For this review, take the finished solid that the model builds, in its own axes (mm). A direction names the side the tool comes from. Coordinates: 2 decimals unless noted, no trailing zeros. Order: outer loops, then holes, each group sorted by start corner. A loop starts at its lowest first (then second) coordinate and runs counter-clockwise, first axis right, second up. Notation, with made-up numbers: (-28.75, 75.25) - (-5.75, 75.25) arc R20 ccw to (-5.75, 112.25) - close; hole circle Ø7 at (38, 11). An arc over 180 degrees is marked (long way). One line per item, written item: value. Start each with the question number.
(1) Consider section A-A on z = -3.25. Write out the cut boundary in (x, y).
(2) Consider section D-D on x = -6.25. Write out the cut boundary in (y, z), then the cut area to 3 significant figures.
(3) Consider section C-C on z = -5.5. Write out the cut boundary in (x, y), then the cut area to 3 significant figures.
(4) Consider section B-B on y = -3.25. Write out the cut boundary in (x, z).
(5) For faces 1 (the flat face through (-7, 3, 6.17)), 2 (the flat face through (0, 0, 10.17)), 3 (the flat face through (-6.825, 1.144, 7.031)), 4 (the flat face through (6.775, 1.144, 7.031)), 5 (the flat face through (0, 2.671, -3)), list the 3-axis set-ups (+Z, -Z, +X, -X, +Y, -Y) from which the entire face can be reached by the end or side of a thin tool; tool diameter is ignored.
(6) To check wall thickness, follow line 1 along X through (y, z) = (-2.5, -6.5); line 2 along X through (y, z) = (2.5, 9); line 3 along Z through (x, y) = (-0.5, 3.75). State the ranges of each line that lie inside material, in increasing order.
(7) Clearance check with flat-ended pins moving along their axes: pin 1 (4 mm diameter, centred on y = 0.5, z = 4, fed in from +X); pin 2 (1 mm diameter, centred on x = -7.5, y = 3, fed in from -Z); pin 3 (8 mm diameter, centred on x = -1.5, z = -6, fed in from -Y). State where each tip first meets the part, or that it passes through.
(8) Mouldability with a two-part tool opening along Y and no side actions: class faces 6 (the flat face through (0, -2.329, -3)), 7 (the flat face through (0, 4.25, 5)), 8 (the flat face through (-3.836, 0, 10)), 9 (the flat face through (0, -1.791, 9)) as released by +Y, released by -Y, zero draft, split by the parting line, or undercut.
```python
from build123d import *

# Parameters (mm, degrees)
SKETCH1_W           = 10
SKETCH1_H           = 8.5
BOSS_EXTRUDE1_DEPTH = 10.67
SKETCH2_W           = 7.4
SKETCH2_H           = 0.5
BOSS_EXTRUDE2_DEPTH = 1.5
SKETCH3_W           = 2.8
SKETCH3_H           = 0.5
BOSS_EXTRUDE3_DEPTH = 7.06
FILLET4_R           = 0.1
SKETCH5_W           = 4.5
SKETCH5_H           = 8.5
BOSS_EXTRUDE4_DEPTH = 3.6
SKETCH6_W           = 4.5
SKETCH6_H           = 8.5
BOSS_EXTRUDE5_DEPTH = 3.6
CUT_EXTRUDE2_START  = -17.2
CUT_EXTRUDE2_DEPTH  = 17.2
BOSS_EXTRUDE6_DEPTH = 10
SKETCH9_W           = 15.5
SKETCH9_H           = 8.5
CUT_EXTRUDE3_DEPTH  = 2
SKETCH10_W          = 7.671768302
SKETCH10_H          = 3.58137051
BOSS_EXTRUDE7_DEPTH = 2
SKETCH12_W          = 7.671768302
SKETCH12_H          = 1.176323548
CUT_EXTRUDE4_DEPTH  = 0.5
FILLET7_R           = 1
FILLET8_R           = 0.5
SKETCH13_W          = 1.4
SKETCH13_H          = 3.317554906
CUT_EXTRUDE5_DEPTH  = 10
FILLET9_R           = 0.3


with BuildPart() as part:
    # Sketch1 → Boss-Extrude1 (new body)
    with BuildSketch(Plane.XY):
        Rectangle(SKETCH1_W, SKETCH1_H)
    extrude(amount=BOSS_EXTRUDE1_DEPTH)

    # Sketch2 → Boss-Extrude2 (add)
    with BuildSketch(Plane(origin=(0, 0, 0), x_dir=(-1, 0, 0), z_dir=(0, 0, -1))):
        with Locations((0.121950207, -2.578749491)):
            Rectangle(SKETCH2_W, SKETCH2_H)
        with Locations((0.121950207, 2.421250509)):
            Rectangle(SKETCH2_W, SKETCH2_H)
    extrude(amount=BOSS_EXTRUDE2_DEPTH)

    # Sketch3 → Boss-Extrude3 (add)
    with BuildSketch(Plane(origin=(0, 0, -1.5), x_dir=(-1, 0, 0), z_dir=(0, 0, -1))):
        with Locations((0, -2.578749491)):
            Rectangle(SKETCH3_W, SKETCH3_H)
        with Locations((0.006424345, 2.421250509)):
            Rectangle(SKETCH3_W, SKETCH3_H)
    extrude(amount=BOSS_EXTRUDE3_DEPTH)

    # Fillet4
    fillet4_edges = [part.edges().sort_by_distance(p)[0] for p in [
        (2.489024896, -2.828749491, -1.5),
        (-2.610975104, -2.328749491, -1.5),
        (-2.614187276, 2.671250509, -1.5),
        (2.485812724, 2.171250509, -1.5),
    ]]
    fillet(fillet4_edges, radius=FILLET4_R)

    # Sketch5 → Boss-Extrude4 (add)
    with BuildSketch(Plane(origin=(5, 0, 0), x_dir=(0, 0, -1), z_dir=(1, 0, 0))):
        with Locations((-8.42, 0)):
            Rectangle(SKETCH5_W, SKETCH5_H)
    extrude(amount=BOSS_EXTRUDE4_DEPTH)

    # Sketch6 → Boss-Extrude5 (add)
    with BuildSketch(Plane.ZY.offset(5)):
        with Locations((8.42, 0)):
            Rectangle(SKETCH6_W, SKETCH6_H)
    extrude(amount=BOSS_EXTRUDE5_DEPTH)

    # Sketch7 → Cut-Extrude2 (cut)
    with BuildSketch(Plane(origin=(8.6, 0, 0), x_dir=(0, 0, -1), z_dir=(1, 0, 0)).offset(CUT_EXTRUDE2_START)):
        Polygon((-6.17, 2.257266115), (-7.916888321, -4.993e-06), (-6.17, -2.262882433), align=None)
    cut_extrude2 = extrude(amount=CUT_EXTRUDE2_DEPTH, mode=Mode.SUBTRACT)

    # Mirror2: Cut-Extrude2 across plane
    add(cut_extrude2.mirror(Plane(origin=(0, 0, 0), x_dir=(0, 0, 1), z_dir=(1, 0, 0))), mode=Mode.SUBTRACT)

    # Sketch8 → Boss-Extrude6 (add)
    with BuildSketch(Plane(origin=(5, 0, 0), x_dir=(0, 0, -1), z_dir=(1, 0, 0))):
        Polygon((-6.17, -2.262882433), (-7.916892176, 0), (-6.17, 2.257266115), align=None)
    extrude(amount=-BOSS_EXTRUDE6_DEPTH)

    # Sketch9 → Cut-Extrude3 (cut)
    with BuildSketch(Plane.XY.offset(10.67)):
        Rectangle(SKETCH9_W, SKETCH9_H)
    extrude(amount=-CUT_EXTRUDE3_DEPTH, mode=Mode.SUBTRACT)

    # Sketch10 → Boss-Extrude7 (add)
    with BuildSketch(Plane.XY.offset(8.67)):
        Rectangle(SKETCH10_W, SKETCH10_H)
    extrude(amount=BOSS_EXTRUDE7_DEPTH)

    # Sketch12 → Cut-Extrude4 (cut)
    with BuildSketch(Plane.XY.offset(10.67)):
        Rectangle(SKETCH12_W, SKETCH12_H)
    extrude(amount=-CUT_EXTRUDE4_DEPTH, mode=Mode.SUBTRACT)

    # Fillet7
    # the kernel refuses this fillet: 1 mm, written as the material it takes off along each edge
    with BuildSketch(Plane(origin=(6.00094766, 0.588161774, 10.67), x_dir=(0, 1, 0), z_dir=(-1, 0, 0))) as fillet7_piece_1:
        with BuildLine():
            CenterArc((0.866025404, 1), FILLET7_R, 210, 60)
            Line((0, 0.5), (-0.017320508, 0.49))
            ThreePointArc((-0.017320508, 0.49), (-0.02, 0.25), (-0.02, 0))
            Line((-0.02, 0), (0, -0.02))
            Line((0, -0.02), (0.866025404, -0.02))
            Line((0.866025404, -0.02), (0.866025404, 0))
        make_face()
    extrude(amount=12.001895321, mode=Mode.SUBTRACT)
    with BuildSketch(Plane(origin=(-6.00094766, -0.588161774, 10.67), x_dir=(0, 0, -1), z_dir=(1, 0, 0))) as fillet7_piece_2:
        with BuildLine():
            CenterArc((1, -0.866025404), FILLET7_R, 120, 60)
            Line((0, -0.866025404), (-0.02, -0.866025404))
            Line((-0.02, -0.866025404), (-0.02, 0))
            Line((-0.02, 0), (0, 0.02))
            ThreePointArc((0, 0.02), (0.25, 0.02), (0.49, 0.017320508))
            Line((0.49, 0.017320508), (0.5, 0))
        make_face()
    extrude(amount=12.001895321, mode=Mode.SUBTRACT)
    with BuildSketch(Plane(origin=(6.335884151, -1.790685255, 10.67), x_dir=(0, 0, -1), z_dir=(-1, 0, 0)), Plane(origin=(-6.335884151, 1.790685255, 10.67), x_dir=(0, 0, -1), z_dir=(1, 0, 0))) as fillet7_piece_3:
        with BuildLine():
            CenterArc((FILLET7_R, -FILLET7_R), FILLET7_R, 90, 90)
            Line((0, -FILLET7_R), (-FILLET7_R * 0.02, -FILLET7_R))
            Line((-FILLET7_R * 0.02, -FILLET7_R), (-FILLET7_R * 0.02, FILLET7_R * 0.02))
            Line((-FILLET7_R * 0.02, FILLET7_R * 0.02), (FILLET7_R, FILLET7_R * 0.02))
            Line((FILLET7_R, FILLET7_R * 0.02), (FILLET7_R, 0))
        make_face()
    extrude(amount=12.671768302, mode=Mode.SUBTRACT)

    # Fillet8
    fillet8_edges = [part.edges().sort_by_distance(p)[0] for p in [
        (0, 1.122436216, 10.613367002),
        (0, -1.122436216, 10.613367002),
    ]]
    fillet(fillet8_edges, radius=FILLET8_R)

    # Sketch13 → Cut-Extrude5 (cut)
    with BuildSketch(Plane(origin=(0, 2.671250509, 0), x_dir=(1, 0, 0), z_dir=(0, 1, 0))):
        with Locations((0, 5.735027383)):
            Rectangle(SKETCH13_W, SKETCH13_H)
    extrude(amount=-CUT_EXTRUDE5_DEPTH, mode=Mode.SUBTRACT)

    # Fillet9
    fillet9_edges = [part.edges().sort_by_distance(p)[0] for p in [
        (0.7, -2.578749491, -7.393804836),
        (0.7, 2.421250509, -7.393804836),
        (0.7, -2.578749491, -4.07624993),
        (0.7, 2.421250509, -4.07624993),
        (-0.7, -2.578749491, -4.07624993),
        (-0.7, 2.421250509, -4.07624993),
        (-0.7, -2.578749491, -7.393804836),
        (-0.7, 2.421250509, -7.393804836),
        (1.4, -2.578749491, -8.56),
        (-1.4, -2.578749491, -8.56),
        (1.393575655, 2.421250509, -8.56),
        (-1.406424345, 2.421250509, -8.56),
    ]]
    fillet(fillet9_edges, radius=FILLET9_R)


solid = part.part
```
Geometry check:
1. outline: (-1.41, 2.17) - (1.39, 2.17) - (1.39, 2.67) - (-1.41, 2.67) - close; (-1.4, -2.83) - (1.4, -2.83) - (1.4, -2.33) - (-1.4, -2.33) - close
2. outline: (-4.25, 6.17) - (-2.26, 6.17) - (0, 7.92) - (2.26, 6.17) - (4.25, 6.17) - (4.25, 8.67) - (-4.25, 8.67) - close
2. area: 17.3 mm^2
3. outline: (-1.41, 2.17) - (-0.7, 2.17) - (-0.7, 2.67) - (-1.41, 2.67) - close; (-1.4, -2.83) - (-0.7, -2.83) - (-0.7, -2.33) - (-1.4, -2.33) - close; (0.7, -2.83) - (1.4, -2.83) - (1.4, -2.33) - (0.7, -2.33) - close; (0.7, 2.17) - (1.39, 2.17) - (1.39, 2.67) - (0.7, 2.67) - close
3. area: 1.40 mm^2
4. outline: (-8.6, 6.17) - (-5, 6.17) - (-5, 0) - (5, 0) - (5, 6.17) - (8.6, 6.17) - (8.6, 10.67) - (7.75, 10.67) - (7.75, 8.67) - (-7.75, 8.67) - (-7.75, 10.67) - (-8.6, 10.67) - close
5. face 1: -Z, -X, +Y, -Y
5. face 2: +Z
5. face 3: -Z, -X
5. face 4: -Z, +X
5. face 5: -Z, +X, -X, +Y
6. line 1: x = -1.4 to -0.7, 0.7 to 1.4
6. line 2: x = -8.6 to -7.75, 7.75 to 8.6
6. line 3: z = 0 to 8.67
7. pin 1: stops at x = 5
7. pin 2: stops at z = 6.17
7. pin 3: stops at y = -2.83
8. face 6: undercut
8. face 7: released by +Y
8. face 8: zero draft
8. face 9: released by -Y
